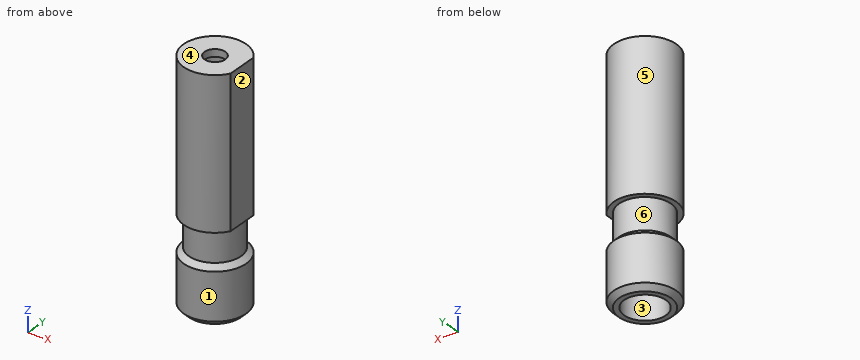
from build123d import *

# Parameters (mm, degrees)
EXTRUDE_1_DEPTH               = 14.2
HOLE_WIZARD_M1_61_D           = 2
HOLE_WIZARD_M1_61_CBORE_D     = 4
HOLE_WIZARD_M1_61_CBORE_DEPTH = 22
CHAMFER_1_SIZE                = 0.5


with BuildPart() as part:
    # Эскиз1 → Бобышка-Вытянуть1 (new body)
    with BuildSketch(Plane(origin=(0, 0, 8.5), x_dir=(-1, 0, 0), z_dir=(0, 0, -1))):
        with BuildLine():
            Line((-2.6, 1.496662955), (-2.6, -1.496662955))
            ThreePointArc((-2.6, -1.496662955), (3, 0), (-2.6, 1.496662955))
        make_face()
    extrude(amount=-EXTRUDE_1_DEPTH)

    # Эскиз2 → Повернуть1 (revolve)
    with BuildSketch(Plane.XZ, mode=Mode.PRIVATE) as revolve_1_sk:
        Polygon((2.5, 8.5), (0, 8.5), (0, 0), (3, 0), (3, 5), (2.5, 5.5), align=None)
    revolve(revolve_1_sk.sketch.rotate(Axis((0, 0, 8.5), (0, 0, -1)), 180), axis=Axis((0, 0, 8.5), (0, 0, -1)))

    # Цековка для винта с внутренним шестигранником M1.61 (through all)
    with Locations(Plane(origin=(0, 0, 0), x_dir=(-1, 0, 0), z_dir=(0, 0, -1))):
        with Locations((0, 0)):
            CounterBoreHole(HOLE_WIZARD_M1_61_D / 2, HOLE_WIZARD_M1_61_CBORE_D / 2, HOLE_WIZARD_M1_61_CBORE_DEPTH)

    # Фаска1
    chamfer_1_edges = [part.edges().sort_by_distance(p)[0] for p in [
        (3, 0, 0),
    ]]
    chamfer(chamfer_1_edges, length=CHAMFER_1_SIZE)


solid = part.part
Model file for the job. Use its own axes, mm. Face numbers are marked on the shaded views. A direction names the side the tool comes from. Round coordinates to 2 decimals unless told otherwise and drop trailing zeros. Loops run counter-clockwise (first coordinate to the right, second up) from the corner with the lowest first, then second, coordinate; pieces in that order, holes last. Notation, with made-up numbers: M 30,39 L 62,39 A24 ccw 62,68 Z; hole C 51.5,31 d11. An arc over 180 degrees is marked long. One line per question, with ' | ' between items.
1) 3-axis set-ups, long thin cutter, end or side, ignore diameter. For the marked faces 1, 2 and 3: which of +Z, -Z, +X, -X, +Y, -Y reach the whole face in a straight line?
Solved:
face 1: +Z, -Z | face 2: +Z, +X, +Y, -Y | face 3: -Z
2) Mould opens along Z. For the marked faces 4, 5 and 6 say: +Z half, -Z half, draft (parallel to the pull), parting line (faces both ways), or undercut.
Solved:
face 4: +Z half | face 5: draft | face 6: undercut
3) Band-saw the part on A-A (y = 0). Give the cut face in (x, z).
Solved:
outline: M -3,0.5 L -2.5,0 L -2,0 L -2,22 L -1,22 L -1,22.7 L -3,22.7 L -3,8.5 L -2.5,8.5 L -2.5,5.5 L -3,5 Z; M 1,22 L 2,22 L 2,0 L 2.5,0 L 3,0.5 L 3,5 L 2.5,5.5 L 2.5,8.5 L 2.6,8.5 L 2.6,22.7 L 1,22.7 Z
4) Flat gauge pins, fed straight in: pin 1 (1.8 mm diameter, centred on x = 0, y = 0, fed in from -Z); pin 2 (1.5 mm diameter, centred on y = 0, z = 18.5, fed in from +X). Where does each tip first touch, or does it go through?
Solved:
pin 1: passes through | pin 2: stops at x = 2.6
5) Drill centre lines: line 1 along Y through (x, z) = (0, 8.75); line 2 along X through (y, z) = (1.5, 21.5); line 3 along X through (y, z) = (1.25, 21.5). Where is each one in solid material? Low to high.
Solved:
line 1: y = -3 to -2, 2 to 3 | line 2: x = -2.6 to -1.32, 1.32 to 2.6 | line 3: x = -2.73 to -1.56, 1.56 to 2.6
6) Band-saw the part on D-D (z = 20.5). Give the cut face in (x, y).
Solved:
outline: M 2.6,-1.5 L 2.6,1.5 A3 ccw long Z; hole C 0,0 d4
7) Band-saw the part on B-B (x = 0). Give the cut face in (y, z).
Solved:
outline: M -3,0.5 L -2.5,0 L -2,0 L -2,22 L -1,22 L -1,22.7 L -3,22.7 L -3,8.5 L -2.5,8.5 L -2.5,5.5 L -3,5 Z; M 1,22 L 2,22 L 2,0 L 2.5,0 L 3,0.5 L 3,5 L 2.5,5.5 L 2.5,8.5 L 3,8.5 L 3,22.7 L 1,22.7 Z
8) Band-saw the part on C-C (z = 1.5). Give the cut face in (x, y).
Solved:
outline: C 0,0 d6; hole C 0,0 d4
